```python
from build123d import *

# Parameters (mm, degrees)
F0_R     = 10
F1_DEPTH = 10


with BuildPart() as f1:
    # F0 (on Front) → F1 (new body)
    with BuildSketch(Plane.XZ):
        with BuildLine():
            ThreePointArc((-5.923694, 24.28806), (-24.821377, -2.983162), (0, -25))
            Line((0, -25), (120, -25))
            Line((120, -25), (120, 55))
            Line((120, 55), (-5.923694, 24.28806))
        make_face()
        Circle(F0_R, mode=Mode.SUBTRACT)
    extrude(amount=F1_DEPTH)


solid = f1.part
```
Source: CAD feature listing. Evaluate the final solid. Frame: model axes, mm. Round coordinates to 2 decimals unless told otherwise and drop trailing zeros. Order: outer loops, then holes, each group sorted by start corner. A loop starts at its lowest first (then second) coordinate and runs counter-clockwise, first axis right, second up. Notation, with made-up numbers: (-26, 78.5) -> (-11, 78.5) arc R12 cw to (-11, 98.5) -> close; hole circle Ø2 at (29.25, 63). An arc over 180 degrees is marked (long way). One line per item, written item: value. Start each with the question number.
Q1. Section query C-C (x = 50). Return the cut outline in (y, z), plus the area to 3 significant figures.
Q2. Pin query (flat end, axial travel): pin 1 (1 mm diameter, centred on x = 12, y = -2.5, fed in from +Z); pin 2 (2 mm diameter, centred on x = 72.5, y = -9, fed in from +Z); pin 3 (6 mm diameter, centred on y = -6.5, z = -1.5, fed in from -X). Return the tip coordinate at first contact, or that it passes through.
Q3. Section query A-A (z = 0). Return the cut outline in (x, y), plus the area to 3 significant figures.
Q4. Section query D-D (z = 45.5). Return the cut outline in (x, y), plus the area to 3 significant figures.
Q5. Material intervals for probe 1 along X at (y, z) = (-5.5, 14); probe 2 along Z at (x, y) = (7.5, -7.75); probe 3 along Z at (x, y) = (-12.5, -2), sorted ascending.
Q6. Section query B-B (y = -4.25). Return the cut outline in (x, z), plus the area to 3 significant figures.
Findings below:
1. outline: (-10, -25) -> (0, -25) -> (0, 37.93) -> (-10, 37.93) -> close
1. area: 629 mm²
2. pin 1: z = 28.78
2. pin 2: z = 43.66
2. pin 3: x = -25
3. outline: (-25, -10) -> (-10, -10) -> (-10, 0) -> (-25, 0) -> close; (10, -10) -> (120, -10) -> (120, 0) -> (10, 0) -> close
3. area: 1,250 mm²
4. outline: (81.05, -10) -> (120, -10) -> (120, 0) -> (81.05, 0) -> close
4. area: 390 mm²
5. probe 1: -20.71 to 120
5. probe 2: -25 to -6.61, 6.61 to 27.56
5. probe 3: -21.65 to 21.65
6. outline: (-5.92, 24.29) arc R25 ccw to (0, -25) -> (120, -25) -> (120, 55) -> close; hole circle Ø20 at (0, 0)
6. area: 8,510 mm²
